Input: part model. Units: mm. Frame: model coordinates. A direction names the side the tool comes from. Coordinates: 2 decimals unless noted, no trailing zeros. Write each loop counter-clockwise with the first axis right and the second up, starting at its lowest first coordinate (ties: lowest second). Pieces come first, ordered by that corner, then holes. Notation, with made-up numbers: (-34.75, 18) - (24.25, 18) arc R17 cw to (24.25, 24) - close; hole circle Ø2 at (-13, 41). An arc over 180 degrees is marked (long way). Use a Markdown table: item, result. Add a question column.
Q1. Set-up query: faces 5 (the face through (55.3, 1.2, -95)), 6 (the face through (110, 12.58, -5)), 7 (the face through (-113.028, 6.202, 3.416)). Return all of +Z, -Z, +X, -X, +Y, -Y with unobstructed straight access to the full face (end or side cutting, diameter ignored); none if empty.
Q2. Pin query (flat end, axial travel): P1, Ø0.7, axis at y = 1.5, z = -8.5, coming from the +X side; P2, Ø10.5, axis at x = -7.5, z = -179.5, coming from the +Y side; P3, Ø1.5, axis at y = 6, z = -126, coming from the +X side. Return the tip coordinate at first contact, or that it passes through.
Q3. Section query D-D (x = 23.5). Return the cut outline in (y, z), then the cut area to 3 significant figures.
Q4. Mould query, pull axis Z, two halves, no side actions, for faces 1 (the face through (-111.248, 6.303, 2.499)), 2 (the face through (-55.6, 15.58, -101.6)), 3 (the face through (42.74, 1.19, -85.16)), 4 (the face through (112.972, 6.202, 3.513)). Classes: released by +Z, released by -Z, zero draft, split by the parting line, or undercut.
Q5. Material intervals for probe 1 along Y at (x, z) = (39, -89); probe 2 along X at (y, z) = (11.5, -17); probe 3 along X at (y, z) = (14.25, -63.5), sorted ascending. Write a range as from..to.
Q6. Section query B-B (x = -85.5). Return the cut outline in (y, z), then the cut area to 3 significant figures.
Q7. Section query A-A (y = 9.75). Return the cut outline in (x, z) (3 decimals).
Q8. Section query C-C (z = -166). Return the cut outline in (x, y), then the cut area to 3 significant figures.
from build123d import *

# Parameters (mm, degrees)
BOSS_EXTRUDE1_DEPTH = 0.2
BOSS_EXTRUDE2_DEPTH = 12.58
SKETCH1_4_W         = 162.49
SKETCH1_4_H         = 2
BOSS_EXTRUDE3_DEPTH = 15.58
BOSS_EXTRUDE5_DEPTH = 2
SKETCH3_7_W         = 160
SKETCH3_7_H         = 15.8
REVOLVE3_ANGLE      = 8
REVOLVE4_ANGLE      = 8


# Read off the part's stored shape, not the designer's step: Boss-Extrude2
with BuildPart() as part:
    # Sketch1 → Boss-Extrude1 (new body)
    with BuildSketch(Plane(origin=(0, 0, 0), x_dir=(1, 0, 0), z_dir=(0, 1, 0))):
        Polygon((-115, 0), (-111, -6.92820323), (111, -6.92820323), (115, 0), (15.625, 172.122549002), (13.892949192, 171.122549002), (2.845299462, 190.25763964), (-2.845299462, 190.25763964), (-13.892949192, 171.122549002), (-15.625, 172.122549002), align=None)
    extrude(amount=BOSS_EXTRUDE1_DEPTH)

    # Boss-Extrude2 outline → Boss-Extrude2 (add)
    with BuildSketch(Plane(origin=(0, 0, 0), x_dir=(1, 0, 0), z_dir=(0, 1, 0))):
        Polygon((15.625, 172.122549002), (4, 192.25763964), (-4, 192.25763964), (-15.625, 172.122549002), (-13.892949192, 171.122549002), (-2.845299462, 190.25763964), (2.845299462, 190.25763964), (13.892949192, 171.122549002), align=None)
        Polygon((62, 91.798692801), (57, 100.458946839), (55.267949192, 99.458946839), (60.267949192, 90.798692801), align=None)
        Polygon((-95.137949192, 30.402081141), (-96.87, 31.402081141), (-115, 0), (-111, -6.92820323), (-74.74, -6.92820323), (-74.74, -4.92820323), (-109.845299462, -4.92820323), (-112.690598923, 0), align=None)
        Polygon((115, 0), (103.375, 20.135090638), (101.642949192, 19.135090638), (112.690598923, 0), (109.845299462, -4.92820323), (87.75, -4.92820323), (87.75, -6.92820323), (111, -6.92820323), align=None)
    extrude(amount=BOSS_EXTRUDE2_DEPTH)

    # Sketch1<4> → Boss-Extrude3 (add)
    with BuildSketch(Plane(origin=(0, 0, 0), x_dir=(1, 0, 0), z_dir=(0, 1, 0))):
        Polygon((-15.625, 172.122549002), (-96.87, 31.402081141), (-95.137949192, 30.402081141), (-13.892949192, 171.122549002), align=None)
        with Locations((6.505, -5.92820323)):
            Rectangle(SKETCH1_4_W, SKETCH1_4_H)
        Polygon((57, 100.458946839), (15.625, 172.122549002), (13.892949192, 171.122549002), (55.267949192, 99.458946839), align=None)
        Polygon((101.642949192, 19.135090638), (103.375, 20.135090638), (62, 91.798692801), (60.267949192, 90.798692801), align=None)
    extrude(amount=BOSS_EXTRUDE3_DEPTH)

    # Sketch3 → Boss-Extrude5 (add)
    with BuildSketch(Plane(origin=(0, 0.2, 0), x_dir=(1, 0, 0), z_dir=(0, 1, 0))):
        Polygon((2.179491924, 155.410852123), (15.862693304, 163.310852123), (95.862693304, 24.746787517), (82.179491924, 16.846787517), align=None)
    extrude(amount=BOSS_EXTRUDE5_DEPTH)

    # Sketch3<7> → Revolve3 (revolve)
    with BuildSketch(Plane(origin=(0, 0.2, 0), x_dir=(1, 0, 0), z_dir=(0, 1, 0))):
        with Locations((0, 5.17179677)):
            Rectangle(SKETCH3_7_W, SKETCH3_7_H)
    revolve(axis=Axis((80, 0.2, -13.07179677), (-1, 0, 0)), revolution_arc=REVOLVE3_ANGLE)

    # Sketch3<8> → Revolve4 (revolve)
    with BuildSketch(Plane(origin=(0, 0.2, 0), x_dir=(1, 0, 0), z_dir=(0, 1, 0))):
        Polygon((-15.862693304, 163.310852123), (-2.179491924, 155.410852123), (-42.179491924, 86.12881982), (-82.179491924, 16.846787517), (-95.862693304, 24.746787517), align=None)
    revolve(axis=Axis((-95.862693304, 0.2, -24.746787517), (-0.500000000000001, 0, 0.866025403784438)), revolution_arc=REVOLVE4_ANGLE)


solid = part.part
Values follow:
| question | item | result |
|---|---|---|
| 1 | face 5 | +Y |
| 1 | face 6 | +Z, +X, +Y |
| 1 | face 7 | +Z, -X, +Y, -Y |
| 2 | P1 | x = 110.29 |
| 2 | P2 | y = 12.58 |
| 2 | P3 | x = 42.69 |
| 3 | outline | (0, -158.48) - (15.58, -158.48) - (15.58, -154.48) - (0.2, -154.48) - (0.2, -150.08) - (2.2, -150.08) - (2.2, -118.48) - (0.2, -118.48) - (0.2, -13.07) - (2.4, 2.57) arc R15.8 ccw to (0.2, 2.73) - (0.2, 4.93) - (15.58, 4.93) - (15.58, 6.93) - (0, 6.93) - close |
| 3 | area | 206 mm2 |
| 4 | face 1 | undercut |
| 4 | face 2 | zero draft |
| 4 | face 3 | undercut |
| 4 | face 4 | released by +Z |
| 5 | probe 1 | 0..0.2 |
| 5 | probe 2 | -105.19..-102.88, 102.88..105.19 |
| 5 | probe 3 | -78.34..-76.03, 76.03..78.34 |
| 6 | outline | (0, -51.1) - (15.58, -51.1) - (15.58, -47.1) - (0.2, -47.1) - (0.2, -42.7) - (1.88, -18.76) - (0.2, -18.76) - (0.2, 4.93) - (12.58, 4.93) - (12.58, 6.93) - (0, 6.93) - close |
| 6 | area | 118 mm2 |
| 7 | outline | (-115, 0) - (-4, -192.258) - (4, -192.258) - (115, 0) - (111, 6.928) - (-111, 6.928) - close; hole (-112.691, 0) - (-2.845, -190.258) - (2.845, -190.258) - (112.691, 0) - (109.845, 4.928) - (-109.845, 4.928) - close |
| 8 | outline | (-19.16, 0) - (19.16, 0) - (19.16, 15.58) - (16.85, 15.58) - (16.85, 0.2) - (-16.85, 0.2) - (-16.85, 15.58) - (-19.16, 15.58) - close |
| 8 | area | 78.7 mm2 |
